from build123d import *

# Parameters (mm, degrees)
PAD_DEPTH    = 21
SKETCH001_R  = 3
POCKET_DEPTH = 3


with BuildPart() as part:
    # Sketch → Pad (new body)
    with BuildSketch(Plane.YZ):
        Polygon((-7.5, 7.1), (-1.5, 0), (0, 0), (0, 7.7), (-3.9, 7.7), (-3.9, 7.1), align=None)
    pad = extrude(amount=PAD_DEPTH)

    # Mirrored: Pad across Sketch V_Axis
    add(pad.mirror(Plane(origin=(0, 0, 0), x_dir=(1, 0, 0), z_dir=(0, 1, 0))))

    # Sketch001 (on Face10 of Mirrored) → Pocket (cut)
    with BuildSketch(Plane(origin=(0, 0, 7.7), x_dir=(0, -1, 0), z_dir=(0, 0, 1))):
        with Locations((0, 5)):
            Circle(SKETCH001_R)
    extrude(amount=-POCKET_DEPTH, mode=Mode.SUBTRACT)


solid = part.part
Here's how the part is built. I have some questions about the finished solid (model axes, mm). A direction names the side the tool comes from. Coordinates: 2 decimals unless noted, no trailing zeros. Loops run counter-clockwise (first coordinate to the right, second up) from the corner with the lowest first, then second, coordinate; pieces in that order, holes last.
1. I need wall thicknesses on L1, parallel to X at y = 0, z = 5.3; L2, parallel to Y at x = 7.5, z = 5.75; L3, parallel to Z at x = 15, y = -2.75. Which ranges of each line are inside material? Lowest first, please.
2. Imagine slicing it at B-B, the plane y = 0. Please give me the cut outline in (x, z).
3. For P1, Ø1, axis at x = 4, z = 3, coming from the -Y side; P2, Ø5, axis at x = 5, y = 0, coming from the +Z side; P3, Ø1.5, axis at x = 11.5, y = -4, coming from the -Z side, each with a flat end and sliding along its axis, tell me the tip position at first contact or that it passes through.
4. If we mould it in two halves opening along Y, with no side actions, what happens to faces 1 (the flat face through (10.35, 4.54, 3.6)), 2 (the flat face through (5, 0, 4.7)), 3 (the flat face through (10, 6, 7.1))? For each: pulls with the +Y half, pulls with the -Y half, needs draft (parallel to the pull), parting line crosses it, or undercut.
5. Imagine slicing it at A-A, the plane x = 5. Please give me the cut outline in (y, z), and give its area (3 significant figures).
6. For faces 4 (the flat face through (21, 0, 5)), 5 (the cylindrical face through (2.07, 0.65, 6.22)), 6 (the flat face through (10, -6, 7.1)), which set-ups out of +Z, -Z, +X, -X, +Y, -Y let a thin tool reach every point of the face, with its end or its side?
7. Imagine slicing it at D-D, the plane x = 15. Please give me the cut outline in (y, z).
8. Imagine slicing it at C-C, the plane z = 6. Please give me the cut outline in (x, y), and give its area (3 significant figures).
Taken from the geometry:
1. L1: x = 0 to 2, 8 to 21
1. L2: y = -6.36 to -1.66, 1.66 to 6.36
1. L3: z = 1.48 to 7.7
2. outline: (0, 0) - (21, 0) - (21, 7.7) - (8, 7.7) - (8, 4.7) - (2, 4.7) - (2, 7.7) - (0, 7.7) - close
3. P1: stops at y = -4.46
3. P2: stops at z = 4.7
3. P3: stops at z = 2.07
4. face 1: pulls with the +Y half
4. face 2: undercut
4. face 3: needs draft
5. outline: (-7.5, 7.1) - (-1.5, 0) - (1.5, 0) - (7.5, 7.1) - (3.9, 7.1) - (3.9, 7.7) - (3, 7.7) - (3, 4.7) - (-3, 4.7) - (-3, 7.7) - (-3.9, 7.7) - (-3.9, 7.1) - close
5. area: 50.6 mm2
6. face 4: +Z, -Z, +X, +Y, -Y
6. face 5: +Z
6. face 6: +Z, +X, -X, -Y
7. outline: (-7.5, 7.1) - (-1.5, 0) - (1.5, 0) - (7.5, 7.1) - (3.9, 7.1) - (3.9, 7.7) - (-3.9, 7.7) - (-3.9, 7.1) - close
8. outline: (0, -6.57) - (21, -6.57) - (21, 6.57) - (0, 6.57) - close; hole circle Ø6 at (5, 0)
8. area: 248 mm2
